Drawing for the job (mm, zero at the part's lowest x, y, z). Round coordinates to 2 decimals unless told otherwise and drop trailing zeros. Write each loop counter-clockwise with the first axis right and the second up, starting at its lowest first coordinate (ties: lowest second). Pieces come first, ordered by that corner, then holes. Notation, with made-up numbers: M -4.75,56.25 L 3.25,56.25 A17 ccw 3.25,60.25 Z; hole C -6,37 d1. An arc over 180 degrees is marked long. Use a Markdown table: item, result.
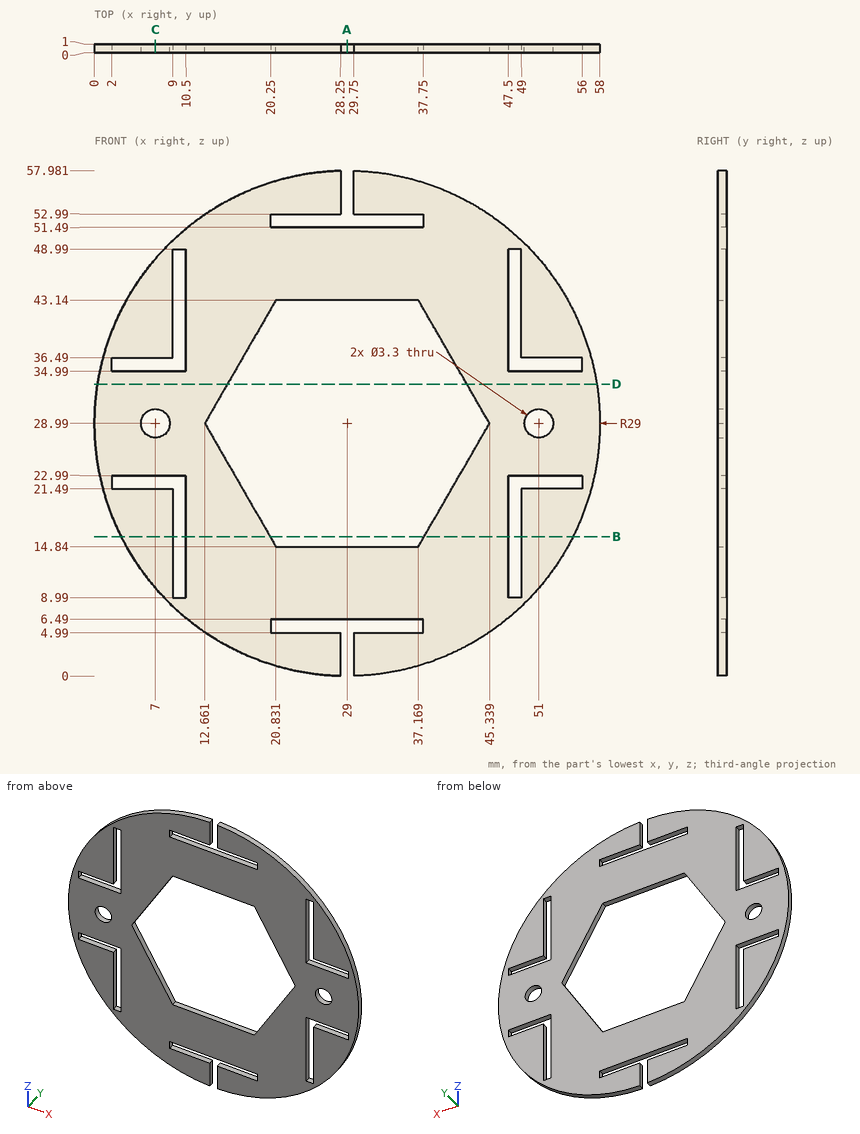
Q1. Cut at B-B on z = 16. Give the cut face in (x, y).
Response values:
| item | result |
|---|---|
| outline | M 3.07,0 L 9,0 L 9,1 L 3.07,1 Z; M 10.5,0 L 20.16,0 L 20.16,1 L 10.5,1 Z; M 37.84,0 L 47.5,0 L 47.5,1 L 37.84,1 Z; M 49,0 L 54.93,0 L 54.93,1 L 49,1 Z |
Q2. Cut at A-A on x = 29. Give the cut face in (y, z).
Response values:
| item | result |
|---|---|
| outline | M 0,6.49 L 1,6.49 L 1,14.84 L 0,14.84 Z; M 0,43.14 L 1,43.14 L 1,51.49 L 0,51.49 Z |
Q3. Drill centre lines: L1, parallel to X at y = 0.9, z = 36; L2, parallel to X at y = 0.65, z = 43.5; L3, parallel to X at y = 0.55, z = 10.5. Where is each one in solid material? Low to high.
Response values:
| item | result |
|---|---|
| L1 | x = 0.86 to 2, 10.5 to 16.71, 41.29 to 47.5, 56 to 57.14 |
| L2 | x = 3.89 to 9, 10.5 to 47.5, 49 to 54.11 |
| L3 | x = 6.66 to 9, 10.5 to 47.5, 49 to 51.34 |
Q4. Drop flat-ended pins along their axis: P1, Ø0.5, axis at y = 0.5, z = 39.5, coming from the -X side (1 decimal); P2, Ø1.5, axis at x = 50, z = 51.5, coming from the +Y side; P3, Ø4, axis at x = 13, z = 43, coming from the -Y side. Give the stop position or say it passes through.
Response values:
| item | result |
|---|---|
| P1 | stops at x = 1.9 |
| P2 | passes through |
| P3 | stops at y = 0 |
Q5. Cut at C-C on x = 7. Give the cut face in (y, z) (1 decimal).
Response values:
| item | result |
|---|---|
| outline | M 0,10.1 L 1,10.1 L 1,21.5 L 0,21.5 Z; M 0,23 L 1,23 L 1,27.3 L 0,27.3 Z; M 0,30.6 L 1,30.6 L 1,35 L 0,35 Z; M 0,36.5 L 1,36.5 L 1,47.9 L 0,47.9 Z |
Q6. Cut at D-D on z = 33.5. Give the cut face in (x, y) (1 decimal).
Response values:
| item | result |
|---|---|
| outline | M 0.4,0 L 15.3,0 L 15.3,1 L 0.4,1 Z; M 42.7,0 L 57.6,0 L 57.6,1 L 42.7,1 Z |
